from build123d import *

# Parameters (mm, degrees)
F1_DEPTH = 15
F2_R     = 25
F3_DEPTH = 20
F5_R     = 75
F6_DEPTH = 25


with BuildPart() as f1:
    # F0 (on Top) → F1 (new body)
    with BuildSketch(Plane.XY):
        with BuildLine():
            ThreePointArc((15, -31.6227766017), (29.5803989155, -18.7082869339), (35, 0))
            ThreePointArc((35, 0), (29.5803989155, 18.7082869339), (15, 31.6227766017))
            Line((15, 31.6227766017), (15, 27.5))
            Line((15, 27.5), (-15, 27.5))
            Line((-15, 27.5), (-15, 31.6227766017))
            ThreePointArc((-15, 31.6227766017), (-35, 0), (-15, -31.6227766017))
            Line((-15, -31.6227766017), (-15, -27.5))
            Line((-15, -27.5), (15, -27.5))
            Line((15, -27.5), (15, -31.6227766017))
        make_face()
        with BuildLine():
            Line((15, 27.5), (15, 31.6227766017))
            ThreePointArc((15, 31.6227766017), (0, 35), (-15, 31.6227766017))
            Line((-15, 31.6227766017), (-15, 27.5))
            Line((-15, 27.5), (15, 27.5))
        make_face()
        with BuildLine():
            ThreePointArc((-15, 31.6227766017), (0, 35), (15, 31.6227766017))
            Line((15, 31.6227766017), (15, 47))
            Line((15, 47), (-15, 47))
            Line((-15, 47), (-15, 31.6227766017))
        make_face()
        with BuildLine():
            Line((15, -47), (15, -31.6227766017))
            ThreePointArc((15, -31.6227766017), (0, -35), (-15, -31.6227766017))
            Line((-15, -31.6227766017), (-15, -47))
            Line((-15, -47), (15, -47))
        make_face()
        with BuildLine():
            ThreePointArc((-15, -31.6227766017), (0, -35), (15, -31.6227766017))
            Line((15, -31.6227766017), (15, -27.5))
            Line((15, -27.5), (-15, -27.5))
            Line((-15, -27.5), (-15, -31.6227766017))
        make_face()
    extrude(amount=F1_DEPTH)

    # F2 (on Top) → F3 (join)
    with BuildSketch(Plane.XY):
        Circle(F2_R)
    extrude(amount=-F3_DEPTH)

    # F5 (on offset) → F6 (join)
    with BuildSketch(Plane.XY.offset(-20)):
        Circle(F5_R)
    extrude(amount=-F6_DEPTH)


solid = f1.part
For this review, take the finished solid that the model builds, in its own axes (mm). A direction names the side the tool comes from. Coordinates: 2 decimals unless noted, no trailing zeros. Write each loop counter-clockwise with the first axis right and the second up, starting at its lowest first coordinate (ties: lowest second). Pieces come first, ordered by that corner, then holes. Notation, with made-up numbers: (9, 0) -> (15, 0) arc R24 ccw to (15, 25) -> close; hole circle Ø9 at (47.5, 60). An arc over 180 degrees is marked (long way). Write each question's results on one line, items separated by ' | '. Start each with the question number.
1) Insertion check: pin 1 (7.5 mm diameter, centred on y = -37, z = 6.5, fed in from +X); pin 2 (4.5 mm diameter, centred on y = 41.5, z = 7.5, fed in from -X); pin 3 (10 mm diameter, centred on x = 21.5, z = -32.5, fed in from -Y); pin 4 (8 mm diameter, centred on x = -18, y = -34, fed in from +Z). Each pin has a flat end and moves straight along its axis. Give the tip position at first contact, or say it passes through.
2) The part is to be moulded in two halves that separate along Z. For faces 1 (the face through (0, 1, 15)), 2 (the face through (-24, -10, 0)), 3 (the face through (-15, -39, 7)), 4 (the face through (23.846, 7.509, -9.86)), say which applies: +Z half, -Z half, draft (parallel to the pull), parting line (faces both ways), or undercut.
3) Consider section B-B (x = 0). Write out the cut boundary in (y, z), plus the area to 3 significant figures.
4) For faces 5 (the face through (15, -39, 7)), 6 (the face through (0, -47, 7)), 7 (the face through (-34.996, 0.553, 7.395)), list the 3-axis set-ups (+Z, -Z, +X, -X, +Y, -Y) from which the entire face can be reached by the end or side of a thin tool; tool diameter is ignored.
5) Consider section D-D (x = -19). Write out the cut boundary in (y, z).
6) Wall thickness on L1, parallel to Z at x = 56, y = 13.5; L2, parallel to Y at x = -56, z = -25.5; L3, parallel to X at y = 25, z = -31: over which ranges is each line inside the solid? List them lowest first. Write a range as [from, to].
7) Consider section A-A (y = -35.5). Write out the cut boundary in (x, z).
8) Consider section C-C (z = 3.5). Write out the cut boundary in (x, y).
Geometry says:
1) pin 1: x = 15 | pin 2: x = -15 | pin 3: y = -73.16 | pin 4: z = 15
2) face 1: +Z half | face 2: undercut | face 3: draft | face 4: undercut
3) outline: (-75, -45) -> (75, -45) -> (75, -20) -> (25, -20) -> (25, 0) -> (47, 0) -> (47, 15) -> (-47, 15) -> (-47, 0) -> (-25, 0) -> (-25, -20) -> (-75, -20) -> close | area: 6,160 mm^2
4) face 5: +Z, +X, -Y | face 6: +Z, +X, -X, -Y | face 7: +Z, -X
5) outline: (-72.55, -45) -> (72.55, -45) -> (72.55, -20) -> (16.25, -20) -> (16.25, 0) -> (29.39, 0) -> (29.39, 15) -> (-29.39, 15) -> (-29.39, 0) -> (-16.25, 0) -> (-16.25, -20) -> (-72.55, -20) -> close
6) L1: [-45, -20] | L2: [-49.89, 49.89] | L3: [-70.71, 70.71]
7) outline: (-66.07, -45) -> (66.07, -45) -> (66.07, -20) -> (-66.07, -20) -> close; (-15, 0) -> (15, 0) -> (15, 15) -> (-15, 15) -> close
8) outline: (-15, -47) -> (15, -47) -> (15, -31.62) arc R35 ccw to (15, 31.62) -> (15, 47) -> (-15, 47) -> (-15, 31.62) arc R35 ccw to (-15, -31.62) -> close
